Model file for the job. Use its own axes, mm. Give positions to 0.01 mm unless a question says otherwise; leave off trailing zeros. Loops run counter-clockwise (first coordinate to the right, second up) from the corner with the lowest first, then second, coordinate; pieces in that order, holes last. Notation, with made-up numbers: (1, 47) - (22, 47) arc R19 ccw to (22, 72) - close; hole circle Ø11 at (77.25, 20.5). An arc over 180 degrees is marked (long way). Use a Markdown table: item, result.
from build123d import *

# Parameters (mm, degrees)
SKETCH_W     = 40
SKETCH_H     = 14
SKETCH_R     = 2.55
PAD_DEPTH    = 6
CHAMFER_SIZE = 2


with BuildPart() as part:
    # Sketch → Pad (new body)
    with BuildSketch(Plane.XY):
        Rectangle(SKETCH_W, SKETCH_H)
        with Locations((-12, 0)):
            Circle(SKETCH_R, mode=Mode.SUBTRACT)
        with Locations((12, 0)):
            Circle(SKETCH_R, mode=Mode.SUBTRACT)
    extrude(amount=PAD_DEPTH)

    # Chamfer
    chamfer_edges = [part.edges().sort_by_distance(p)[0] for p in [
        (-14.55, 0, 6),
        (9.45, 0, 6),
    ]]
    chamfer(chamfer_edges, length=CHAMFER_SIZE)


solid = part.part
(1) Slice it at A-A, the plane y = 0. Write the cut outline in (x, z).
Computed:
| item | result |
|---|---|
| outline | (-20, 0) - (-14.55, 0) - (-14.55, 4) - (-16.55, 6) - (-20, 6) - close; (-9.45, 0) - (9.45, 0) - (9.45, 4) - (7.45, 6) - (-7.45, 6) - (-9.45, 4) - close; (14.55, 0) - (20, 0) - (20, 6) - (16.55, 6) - (14.55, 4) - close |
(2) Slice it at D-D, the plane z = 4.5. Write the cut outline in (x, y), plus the area to 3 significant figures.
Computed:
| item | result |
|---|---|
| outline | (-20, -7) - (20, -7) - (20, 7) - (-20, 7) - close; hole circle Ø6.1 at (-12, 0); hole circle Ø6.1 at (12, 0) |
| area | 502 mm² |
(3) Slice it at C-C, the plane z = 1.05. Write the cut outline in (x, y), plus the area to 3 significant figures.
Computed:
| item | result |
|---|---|
| outline | (-20, -7) - (20, -7) - (20, 7) - (-20, 7) - close; hole circle Ø5.1 at (-12, 0); hole circle Ø5.1 at (12, 0) |
| area | 519 mm² |
(4) Slice it at B-B, the plane x = -12. Write the cut outline in (y, z).
Computed:
| item | result |
|---|---|
| outline | (-7, 0) - (-2.55, 0) - (-2.55, 4) - (-4.55, 6) - (-7, 6) - close; (2.55, 0) - (7, 0) - (7, 6) - (4.55, 6) - (2.55, 4) - close |
(5) Mould opens along Y. For faces 1 (the flat face through (0, -7, 3)), 2 (the cylindrical face through (-14.024, -1.552, 1.972)), 3 (the flat face through (20, 0, 3)) say: pulls with the +Y half, pulls with the -Y half, needs draft (parallel to the pull), parting line crosses it, or undercut.
Computed:
| item | result |
|---|---|
| face 1 | pulls with the -Y half |
| face 2 | undercut |
| face 3 | needs draft |
(6) Pin check, flat tips, straight feed: P1, Ø2, axis at x = 4, y = -1.5, coming from the -Z side; P2, Ø6.5, axis at x = 12, y = 0, coming from the +Z side. Stop position of each tip, or through.
Computed:
| item | result |
|---|---|
| P1 | z = 0 |
| P2 | z = 4.7 |
(7) Drill centre lines: probe 1 along Y at (x, z) = (-12, 1.8); probe 2 along X at (y, z) = (0.25, 1.55); probe 3 along X at (y, z) = (-0.75, 4). Where is each one in solid material? Low to high. Write a range as [from, to].
Computed:
| item | result |
|---|---|
| probe 1 | [-7, -2.55], [2.55, 7] |
| probe 2 | [-20, -14.54], [-9.46, 9.46], [14.54, 20] |
| probe 3 | [-20, -14.44], [-9.56, 9.56], [14.44, 20] |
